Model file for the job. Use its own axes, mm. Give positions to 0.01 mm unless a question says otherwise; leave off trailing zeros. Write each loop counter-clockwise with the first axis right and the second up, starting at its lowest first coordinate (ties: lowest second). Pieces come first, ordered by that corner, then holes. Notation, with made-up numbers: (40.25, 57) - (63.25, 57) arc R16 cw to (63.25, 85) - close; hole circle Ø8 at (66, -34.75). An arc over 180 degrees is marked (long way). One line per item, written item: value. Start each with the question number.
(1) Cut at B-B, the plane y = 2.9. State how many separate pieces and enclosed holes the cut face has, and give its area (3 significant figures).
(2) Probe L1, parallel to X at y = 4.5, z = -52; L2, parallel to Z at x = 54, y = 2.75 (3 decimals); L3, parallel to X at y = 1.7, z = -56.5. List the from-to ranges inside material, lowest first.
(3) Cut at A-A, the plane z = 36. List the corners of the cut face in (x, y).
from build123d import *

# Parameters (mm, degrees)
SKETCH2_W           = 200
SKETCH2_H           = 185
BOSS_EXTRUDE1_DEPTH = 5
SKETCH3_R           = 1.5
CUT_EXTRUDE1_DEPTH  = 137.313058802
SKETCH4_R           = 1.5
CUT_EXTRUDE3_DEPTH  = 137.313058802
FILLET1_R           = 8


with BuildPart() as part:
    # Sketch2 → Boss-Extrude1 (new body)
    with BuildSketch(Plane(origin=(0, 0, 0), x_dir=(1, 0, 0), z_dir=(0, 1, 0))):
        Rectangle(SKETCH2_W, SKETCH2_H)
        with BuildLine():
            Line((-95, 55.5), (-95, 82.5))
            ThreePointArc((-95, 82.5), (-93.5, 84), (-92, 82.5))
            Line((-92, 82.5), (-92, 55.5))
            ThreePointArc((-92, 55.5), (-93.5, 54), (-95, 55.5))
        make_face(mode=Mode.SUBTRACT)
        with BuildLine():
            Line((95, 55.5), (95, 82.5))
            ThreePointArc((95, 82.5), (93.5, 84), (92, 82.5))
            Line((92, 82.5), (92, 55.5))
            ThreePointArc((92, 55.5), (93.5, 54), (95, 55.5))
        make_face(mode=Mode.SUBTRACT)
        with BuildLine():
            Line((95, -55.5), (95, -82.5))
            ThreePointArc((95, -82.5), (93.5, -84), (92, -82.5))
            Line((92, -82.5), (92, -55.5))
            ThreePointArc((92, -55.5), (93.5, -54), (95, -55.5))
        make_face(mode=Mode.SUBTRACT)
        with BuildLine():
            Line((-95, -55.5), (-95, -82.5))
            ThreePointArc((-95, -82.5), (-93.5, -84), (-92, -82.5))
            Line((-92, -82.5), (-92, -55.5))
            ThreePointArc((-92, -55.5), (-93.5, -54), (-95, -55.5))
        make_face(mode=Mode.SUBTRACT)
    extrude(amount=BOSS_EXTRUDE1_DEPTH)

    # Sketch3 → Cut-Extrude1 (cut, through all)
    with BuildSketch(Plane(origin=(0, 5, 0), x_dir=(1, 0, 0), z_dir=(0, 1, 0))):
        with BuildLine():
            Line((-82.5, 42.5), (-42.5, 42.5))
            ThreePointArc((-42.5, 42.5), (-40, 45), (-42.5, 47.5))
            Line((-42.5, 47.5), (-82.5, 47.5))
            ThreePointArc((-82.5, 47.5), (-85, 45), (-82.5, 42.5))
        make_face()
        with BuildLine():
            ThreePointArc((-42.5, -42.5), (-40, -45), (-42.5, -47.5))
            Line((-42.5, -47.5), (-82.5, -47.5))
            ThreePointArc((-82.5, -47.5), (-85, -45), (-82.5, -42.5))
            Line((-82.5, -42.5), (-42.5, -42.5))
        make_face()
        with Locations(Location((-90, -30, 0), (0, 0, 270))):
            Circle(SKETCH3_R)
        with Locations(Location((-90, 30, 0), (0, 0, 90))):
            Circle(SKETCH3_R)
        with Locations(Location((-35, -30, 0), (0, 0, 90))):
            Circle(SKETCH3_R)
        with Locations(Location((-35, 30, 0), (0, 0, 270))):
            Circle(SKETCH3_R)
    extrude(amount=-CUT_EXTRUDE1_DEPTH, mode=Mode.SUBTRACT)

    # Sketch4 → Cut-Extrude3 (cut, through all)
    with BuildSketch(Plane(origin=(0, 5, 0), x_dir=(1, 0, 0), z_dir=(0, 1, 0))):
        with Locations(Location((8, 46.935, 0), (0, 0, 270))):
            Circle(SKETCH4_R)
        with Locations(Location((52, 46.935, 0), (0, 0, 90))):
            Circle(SKETCH4_R)
        with Locations(Location((6, -46.935, 0), (0, 0, 270))):
            Circle(SKETCH4_R)
        with Locations(Location((54, -46.935, 0), (0, 0, 90))):
            Circle(SKETCH4_R)
        with BuildLine():
            Line((71.5, -60), (71.5, 60))
            ThreePointArc((71.5, 60), (74, 62.5), (76.5, 60))
            Line((76.5, 60), (76.5, -60))
            ThreePointArc((76.5, -60), (74, -62.5), (71.5, -60))
        make_face()
        with BuildLine():
            Line((-16.5, -60), (-16.5, 60))
            ThreePointArc((-16.5, 60), (-14, 62.5), (-11.5, 60))
            Line((-11.5, 60), (-11.5, -60))
            ThreePointArc((-11.5, -60), (-14, -62.5), (-16.5, -60))
        make_face()
        with BuildLine():
            Line((0, 69.435), (60, 69.435))
            ThreePointArc((60, 69.435), (62.5, 66.935), (60, 64.435))
            Line((60, 64.435), (0, 64.435))
            ThreePointArc((0, 64.435), (-2.5, 66.935), (0, 69.435))
        make_face()
        with BuildLine():
            Line((0, -69.435), (60, -69.435))
            ThreePointArc((60, -69.435), (62.5, -66.935), (60, -64.435))
            Line((60, -64.435), (0, -64.435))
            ThreePointArc((0, -64.435), (-2.5, -66.935), (0, -69.435))
        make_face()
    extrude(amount=-CUT_EXTRUDE3_DEPTH, mode=Mode.SUBTRACT)

    # Fillet1
    fillet1_edges = [part.edges().sort_by_distance(p)[0] for p in [
        (100, 2.5, 92.5),
        (-100, 2.5, 92.5),
        (-100, 2.5, -92.5),
        (100, 2.5, -92.5),
    ]]
    fillet(fillet1_edges, radius=FILLET1_R)


solid = part.part
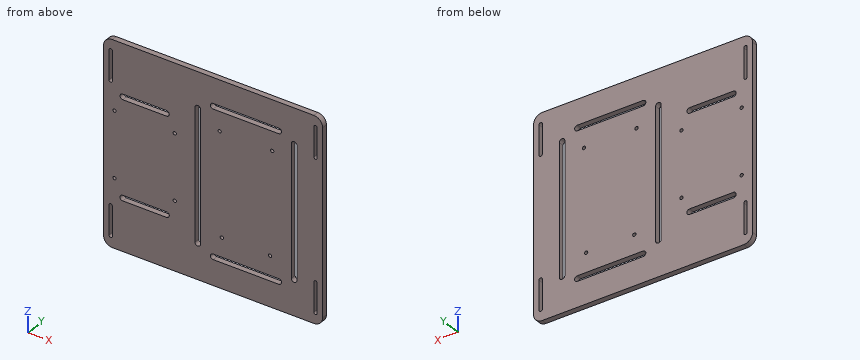
Answers follow:
1. separate pieces: 1
1. enclosed holes: 18
1. area: 34,200 mm²
2. L1: x = -100 to -16.5, -11.5 to 71.5, 76.5 to 100
2. L2: z = -92.5 to -69.435, -64.435 to 45.435, 48.435 to 64.435, 69.435 to 92.5
2. L3: x = -100 to -95, -92 to -16.5, -11.5 to 71.5, 76.5 to 92, 95 to 100
3. outline: (-100, 0) - (-16.5, 0) - (-16.5, 5) - (-100, 5) - close; (-11.5, 0) - (71.5, 0) - (71.5, 5) - (-11.5, 5) - close; (76.5, 0) - (100, 0) - (100, 5) - (76.5, 5) - close
